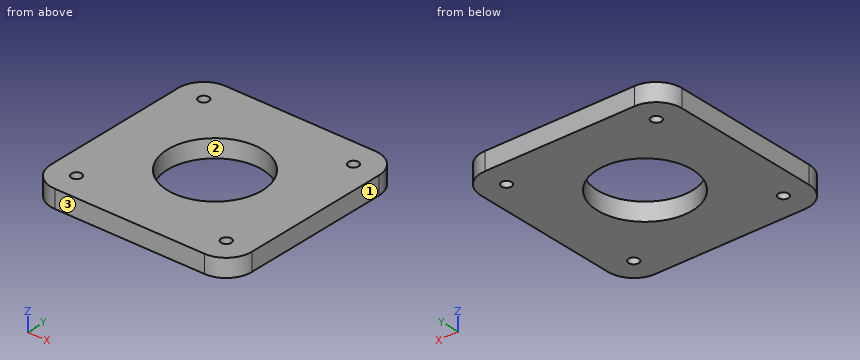
```python
from build123d import *

# Parameters (mm, degrees)
SKETCH1_W           = 78.5
SKETCH1_H           = 78.5
BOSS_EXTRUDE1_DEPTH = 3.5
FILLET1_R           = 10
SKETCH2_R           = 2
CUT_EXTRUDE1_DEPTH  = 56.947520052
SKETCH3_R           = 18.5
CUT_EXTRUDE2_DEPTH  = 56.947520052


with BuildPart() as part:
    # Sketch1 → Boss-Extrude1 (new, symmetric)
    with BuildSketch(Plane.XY):
        Rectangle(SKETCH1_W, SKETCH1_H)
    extrude(amount=BOSS_EXTRUDE1_DEPTH, both=True)

    # Fillet1
    fillet1_edges = [part.edges().sort_by_distance(p)[0] for p in [
        (39.25, -39.25, 0),
        (-39.25, -39.25, 0),
        (-39.25, 39.25, 0),
        (39.25, 39.25, 0),
    ]]
    fillet(fillet1_edges, radius=FILLET1_R)

    # Sketch2 → Cut-Extrude1 (cut, through all)
    with BuildSketch(Plane.XY.offset(3.5)):
        with Locations((-29.25, 29.25)):
            Circle(SKETCH2_R)
        with Locations(Location((-29.25, -29.25, 0), (0, 0, 180))):
            Circle(SKETCH2_R)
        with Locations(Location((29.25, 29.25, 0), (0, 0, 180))):
            Circle(SKETCH2_R)
        with Locations((29.25, -29.25)):
            Circle(SKETCH2_R)
    extrude(amount=-CUT_EXTRUDE1_DEPTH, mode=Mode.SUBTRACT)

    # Sketch3 → Cut-Extrude2 (cut, through all)
    with BuildSketch(Plane.XY.offset(3.5)):
        Circle(SKETCH3_R)
    extrude(amount=-CUT_EXTRUDE2_DEPTH, mode=Mode.SUBTRACT)


solid = part.part
```
Verification items for the finished model (mm, model axes). Face numbers are marked on the shaded views. Give positions to 0.01 mm unless a question says otherwise; leave off trailing zeros. Order: outer loops, then holes, each group sorted by start corner. A loop starts at its lowest first (then second) coordinate and runs counter-clockwise, first axis right, second up. Notation, with made-up numbers: M 56.25,20 L 102.25,20 A7 ccw 102.25,28 Z; hole C -3.5,53.5 d4. An arc over 180 degrees is marked long. Answer in a Markdown table with one row per item. Add a question column.
Item 1: Gauge pin test, flat end, axial feed: pin 1 (3 mm diameter, centred on x = 29.25, y = -29.25, fed in from -Z). Record the tip position at first contact, or that the pin passes through.
Item 2: Mould release check, pull along Y, two halves, no side actions. Record for the marked faces 1, 2 and 3: released by +Y, released by -Y, zero draft, split by the parting line, or undercut.
Item 3: Section check C-C, the plane x = 3. Enter the section's corners in (y, z), and give its area (3 significant figures).
Item 4: Section check B-B, the plane y = 0. Enter the section's corners in (x, z).
Item 5: Section check D-D, the plane y = 34. Enter the section's corners in (x, z).
Item 6: Section check A-A, the plane z = 1. Enter the section's corners in (x, y).
Item 7: Scan lines: probe 1 along Y at (x, z) = (29.25, 0.25); probe 2 along Y at (x, z) = (0, 1); probe 3 along Y at (x, z) = (28.5, 2.75). Record each from-to range of solid material in increasing order. Write a range as from..to.
Filled sheet:
| question | item | result |
|---|---|---|
| 1 | pin 1 | passes through |
| 2 | face 1 | zero draft |
| 2 | face 2 | undercut |
| 2 | face 3 | released by -Y |
| 3 | outline | M -39.25,-3.5 L -18.26,-3.5 L -18.26,3.5 L -39.25,3.5 Z; M 18.26,-3.5 L 39.25,-3.5 L 39.25,3.5 L 18.26,3.5 Z |
| 3 | area | 294 mm^2 |
| 4 | outline | M -39.25,-3.5 L -18.5,-3.5 L -18.5,3.5 L -39.25,3.5 Z; M 18.5,-3.5 L 39.25,-3.5 L 39.25,3.5 L 18.5,3.5 Z |
| 5 | outline | M -38.05,-3.5 L 38.05,-3.5 L 38.05,3.5 L -38.05,3.5 Z |
| 6 | outline | M -39.25,-29.25 A10 ccw -29.25,-39.25 L 29.25,-39.25 A10 ccw 39.25,-29.25 L 39.25,29.25 A10 ccw 29.25,39.25 L -29.25,39.25 A10 ccw -39.25,29.25 Z; hole C -29.25,-29.25 d4; hole C -29.25,29.25 d4; hole C 0,0 d37; hole C 29.25,-29.25 d4; hole C 29.25,29.25 d4 |
| 7 | probe 1 | y = -39.25..-31.25, -27.25..27.25, 31.25..39.25 |
| 7 | probe 2 | y = -39.25..-18.5, 18.5..39.25 |
| 7 | probe 3 | y = -39.25..-31.1, -27.4..27.4, 31.1..39.25 |
